```python
from build123d import *

# Parameters (mm, degrees)
F0_W      = 34.45
F0_H      = 25.1
F1_DEPTH  = 50.65
F2_T      = -3
F3_R      = 4
F3_R_2    = 0.925
F4_DEPTH  = 25
F5_W      = 31.45
F5_H      = 44.65
F6_DEPTH  = 25.101
F7_R      = 8
F8_R      = 6
F9_R      = 0.925
F10_DEPTH = 50.651


with BuildPart() as f1:
    # F0 (on Top) → F1 (new body)
    with BuildSketch(Plane.XY):
        with Locations((1.9014209259, 12.55)):
            Rectangle(F0_W, F0_H)
    extrude(amount=F1_DEPTH)

    # F2
    f2_openings = [f1.faces().sort_by_distance(p)[0] for p in [
        (-15.323579, 12.55, 25.325),
    ]]
    offset(amount=F2_T, openings=f2_openings)

    # F3 (on face) → F4 (cut)
    with BuildSketch(Plane.YZ.offset(19.1264209259)):
        with Locations((12.55, 25.325)):
            Circle(F3_R)
        with Locations((12.55, 17.475)):
            Circle(F3_R_2)
        with Locations((18.1007882323, 19.7742117677)):
            Circle(F3_R_2)
        with Locations((20.4, 25.325)):
            Circle(F3_R_2)
        with Locations((18.1007882323, 30.8757882323)):
            Circle(F3_R_2)
        with Locations((12.55, 33.175)):
            Circle(F3_R_2)
        with Locations((6.9992117677, 30.8757882323)):
            Circle(F3_R_2)
        with Locations((4.7, 25.325)):
            Circle(F3_R_2)
        with Locations((6.9992117677, 19.7742117677)):
            Circle(F3_R_2)
    extrude(amount=-F4_DEPTH, mode=Mode.SUBTRACT)

    # F5 (on face) → F6 (cut, through all)
    with BuildSketch(Plane(origin=(0, 25.1, 0), x_dir=(-1, 0, 0), z_dir=(0, 1, 0))):
        with Locations((-0.4014209259, 25.325)):
            Rectangle(F5_W, F5_H)
    extrude(amount=-F6_DEPTH, mode=Mode.SUBTRACT)

    # F7
    f7_edges = [f1.edges().sort_by_distance(p)[0] for p in [
        (16.126421, 12.55, 47.65),
        (16.126421, 12.55, 3),
    ]]
    fillet(f7_edges, radius=F7_R)

    # F8
    f8_edges = [f1.edges().sort_by_distance(p)[0] for p in [
        (19.126421, 12.55, 50.65),
        (19.126421, 12.55, 0),
    ]]
    fillet(f8_edges, radius=F8_R)

    # F9 (on face) → F10 (cut, through all)
    with BuildSketch(Plane.XY.offset(50.65)):
        with Locations((-10.2235790741, 19.65)):
            Circle(F9_R)
        with Locations((-10.2235790741, 5.45)):
            Circle(F9_R)
        with BuildLine():
            Line((-4.0485790741, 12.55), (-2.1985790741, 12.55))
            ThreePointArc((-2.1985790741, 12.55), (-3.1235790741, 13.475), (-4.0485790741, 12.55))
        make_face()
        with BuildLine():
            ThreePointArc((-4.0485790741, 12.55), (-3.1235790741, 11.625), (-2.1985790741, 12.55))
            Line((-2.1985790741, 12.55), (-4.0485790741, 12.55))
        make_face()
        with BuildLine():
            ThreePointArc((-10.2235790741, 16.55), (-13.0520061988, 15.3784271247), (-14.2235790741, 12.55))
            Line((-14.2235790741, 12.55), (-6.2235790741, 12.55))
            ThreePointArc((-6.2235790741, 12.55), (-7.3951519493, 15.3784271247), (-10.2235790741, 16.55))
        make_face()
        with BuildLine():
            ThreePointArc((-14.2235790741, 12.55), (-13.0520061988, 9.7215728753), (-10.2235790741, 8.55))
            ThreePointArc((-10.2235790741, 8.55), (-7.3951519493, 9.7215728753), (-6.2235790741, 12.55))
            Line((-6.2235790741, 12.55), (-14.2235790741, 12.55))
        make_face()
        with BuildLine():
            Line((-15.3235790741, 16.55), (-15.3235790741, 12.55))
            Line((-15.3235790741, 12.55), (-14.2235790741, 12.55))
            ThreePointArc((-14.2235790741, 12.55), (-13.0520061988, 15.3784271247), (-10.2235790741, 16.55))
            Line((-10.2235790741, 16.55), (-15.3235790741, 16.55))
        make_face()
        with BuildLine():
            Line((-15.3235790741, 12.55), (-15.3235790741, 8.55))
            Line((-15.3235790741, 8.55), (-10.2235790741, 8.55))
            ThreePointArc((-10.2235790741, 8.55), (-13.0520061988, 9.7215728753), (-14.2235790741, 12.55))
            Line((-14.2235790741, 12.55), (-15.3235790741, 12.55))
        make_face()
    extrude(amount=-F10_DEPTH, mode=Mode.SUBTRACT)


solid = f1.part
```
Source: CAD feature listing. Evaluate the final solid. Frame: model axes, mm. A direction names the side the tool comes from. Coordinates: 2 decimals unless noted, no trailing zeros. Loops run counter-clockwise (first coordinate to the right, second up) from the corner with the lowest first, then second, coordinate; pieces in that order, holes last. Notation, with made-up numbers: M 71.5,64 L 79.5,64 A12 ccw 79.5,80 Z; hole C -21.5,18 d4. An arc over 180 degrees is marked long. Use a Markdown table: item, result. Add a question column.
Q1. Material intervals for L1, parallel to Z at x = -7.5, y = 7.25; L2, parallel to Z at x = 17.85, y = 12.55 (3 decimals); L3, parallel to X at y = 14.75, z = 39, sorted ascending.
Q2. Section query B-B, the plane x = -12.5. Return loops of the section in (y, z).
Q3. Section query C-C, the plane x = -7.5. Return loops of the section in (y, z), and give its area (3 significant figures).
Q4. First-contact query: pin 1 (2 mm diameter, centred on x = -10.22, y = 19.65, fed in from -Z); pin 2 (1.5 mm diameter, centred on y = 4.7, z = 25.325, fed in from +X); pin 3 (3 mm diameter, centred on y = 12.55, z = 17.475, fed in from -X). Flat tips, straight axial feed; report the tip coordinate or a pass-through.
Q5. Section query A-A, the plane x = 1. Return loops of the section in (y, z), and give its area (3 significant figures).
Q6. Draft query along X for faces 4 (the flat face through (19.126, 12, 21)), 5 (the flat face through (16.126, 16, 22)), 6 (the cylindrical face through (-2.923, 13.453, 49.171)), 7 (the cylindrical face through (17.647, 13.404, 32.821)). Return one class per face: pulls with the +X half, pulls with the -X half, needs draft (parallel to the pull), parting line crosses it, or undercut.
Q7. Access query for faces 1 (the cylindrical face through (13.72, 12.37, 5.28)), 2 (the cylindrical face through (-9.797, 18.829, 1.521)), 3 (the flat face through (-13, 8.55, 2)). Directions: +Z, -Z, +X, -X, +Y, -Y. A direction counts if a zero-diameter tool reaches every point of the face in a straight line with its end or side. Return the directions, or none.
Q8. Section query D-D, the plane z = 12. Return loops of the section in (x, y), and give its area (3 significant figures).
Result:
| question | item | result |
|---|---|---|
| 1 | L1 | z = 0 to 3, 47.65 to 50.65 |
| 1 | L2 | z = 2.3 to 16.55, 18.4 to 21.325, 29.325 to 32.25, 34.1 to 48.35 |
| 1 | L3 | x = 16.13 to 19.13 |
| 2 | outline | M 0,0 L 8.55,0 L 8.55,3 L 0,3 Z; M 0,47.65 L 8.55,47.65 L 8.55,50.65 L 0,50.65 Z; M 16.55,0 L 25.1,0 L 25.1,3 L 16.55,3 Z; M 16.55,47.65 L 25.1,47.65 L 25.1,50.65 L 16.55,50.65 Z |
| 3 | outline | M 0,0 L 9.62,0 L 9.62,3 L 0,3 Z; M 0,47.65 L 9.62,47.65 L 9.62,50.65 L 0,50.65 Z; M 15.48,0 L 25.1,0 L 25.1,3 L 15.48,3 Z; M 15.48,47.65 L 25.1,47.65 L 25.1,50.65 L 15.48,50.65 Z |
| 3 | area | 115 mm2 |
| 4 | pin 1 | stops at z = 0 |
| 4 | pin 2 | passes through |
| 4 | pin 3 | stops at x = 16.13 |
| 5 | outline | M 0,0 L 25.1,0 L 25.1,3 L 0,3 Z; M 0,47.65 L 25.1,47.65 L 25.1,50.65 L 0,50.65 Z |
| 5 | area | 151 mm2 |
| 6 | face 4 | pulls with the +X half |
| 6 | face 5 | pulls with the -X half |
| 6 | face 6 | undercut |
| 6 | face 7 | needs draft |
| 7 | face 1 | -X, +Y, -Y |
| 7 | face 2 | +Z, -Z |
| 7 | face 3 | +Z, -Z, -X |
| 8 | outline | M 16.13,0 L 19.13,0 L 19.13,25.1 L 16.13,25.1 Z |
| 8 | area | 75.3 mm2 |
